Can you work these out from the drawing? Everything is in mm from the part's minimum corner. A direction names the side the tool comes from. Round coordinates to 2 decimals unless told otherwise and drop trailing zeros. Write each loop counter-clockwise with the first axis right and the second up, starting at its lowest first coordinate (ties: lowest second). Pieces come first, ordered by that corner, then holes. Notation, with made-up numbers: (18, 47.25) -> (26, 47.25) arc R3 ccw to (26, 52.25) -> close; hole circle Ø6 at (-23, 35). An arc over 180 degrees is marked (long way). Write item = value, one per line. Start each with the question number.
1) Imagine slicing it at B-B, the plane y = 18. Please give me the cut outline in (x, z).
2) Imagine slicing it at D-D, the plane y = 7. Please give me the cut outline in (x, z).
3) Imagine slicing it at A-A, the plane z = 2. Please give me the cut outline in (x, y) (1 decimal), then the cut area to 3 significant figures.
4) For the marked faces 4, 5 and 6, which set-ups out of +Z, -Z, +X, -X, +Y, -Y let a thin tool reach every point of the face, with its end or its side?
5) Thinking about a two-plate mould opening in Y: for the marked faces 1, 2 and 3, which applies, +Y half, -Y half, draft (parallel to the pull), parting line (faces both ways), or undercut?
6) I'm going to push flat-ended pins straight in: pin 1 (8.5 mm diameter, centred on x = 14.5, y = 5, fed in from +Z); pin 2 (3 mm diameter, centred on y = 22.5, z = 2.5, fed in from -X); pin 3 (1.5 mm diameter, centred on x = 30.5, z = 9, fed in from -Y). Where does each tip first touch, or does it pass through?
7) If I drill on line 1 (Y direction, x = 24, z = 6); line 2 (Z direction, x = 25, y = 40); line 3 (Y direction, x = 18, z = 5.75), over which ranges is the centre line in solid material (lowest first)?
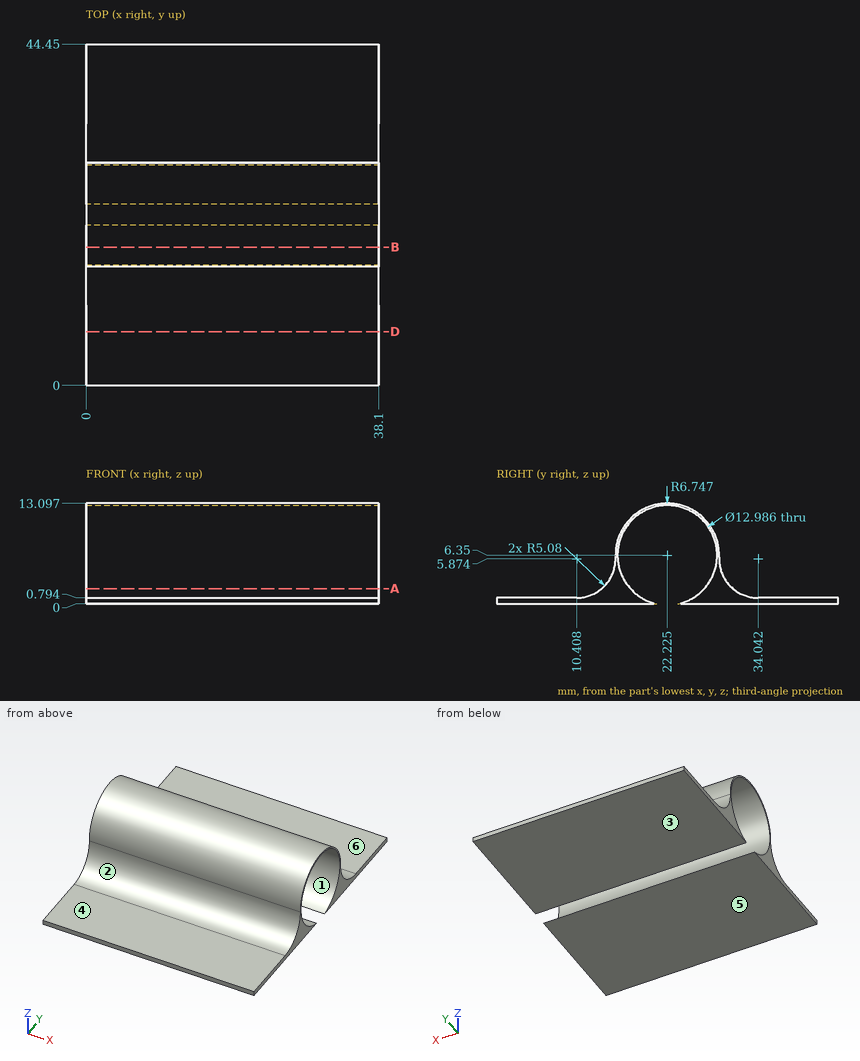
Reported:
q1.outline = (0, 0) -> (38.1, 0) -> (38.1, 1.42) -> (0, 1.42) -> close; (0, 11.28) -> (38.1, 11.28) -> (38.1, 11.61) -> (0, 11.61) -> close
q2.outline = (0, 0) -> (38.1, 0) -> (38.1, 0.79) -> (0, 0.79) -> close
q3.outline = (0, 13.7) -> (38.1, 13.7) -> (38.1, 17.4) -> (0, 17.4) -> close; (0, 27) -> (38.1, 27) -> (38.1, 30.8) -> (0, 30.8) -> close
q3.area = 283 mm²
q4.face_4 = +Z, +X, -X, -Y
q4.face_5 = -Z, +X, -X, +Y, -Y
q4.face_6 = +Z, +X, -X, +Y
q5.face_1 = undercut
q5.face_2 = -Y half
q5.face_3 = draft
q6.pin_1 = 0.79
q6.pin_2 = through
q6.pin_3 = 15.75
q7.line_1 = 15.49 to 15.74, 28.71 to 28.96
q7.line_2 = 0 to 0.79
q7.line_3 = 15.49 to 15.76, 28.69 to 28.96
